For this review, take the finished solid that the model builds, in its own axes (mm). Give positions to 0.01 mm unless a question says otherwise; leave off trailing zeros. Loops run counter-clockwise (first coordinate to the right, second up) from the corner with the lowest first, then second, coordinate; pieces in that order, holes last. Notation, with made-up numbers: (-26.75, 21) - (-14.75, 21) arc R10 cw to (-14.75, 37) - close; hole circle Ø3 at (-23, 31.5). An arc over 180 degrees is marked (long way). Answer in a Markdown table with one row per item.
```python
from build123d import *

# Parameters (mm, degrees)
F0_W     = 21
F0_H     = 21
F1_DEPTH = 680
F3_DEPTH = 12.5


with BuildPart() as f1:
    # F0 (on Top) → F1 (new body)
    with BuildSketch(Plane.XY):
        with BuildLine():
            ThreePointArc((12.5, 9.5), (11.62132, 11.62132), (9.5, 12.5))
            Line((9.5, 12.5), (-9.5, 12.5))
            ThreePointArc((-9.5, 12.5), (-11.62132, 11.62132), (-12.5, 9.5))
            Line((-12.5, 9.5), (-12.5, -9.5))
            ThreePointArc((-12.5, -9.5), (-11.62132, -11.62132), (-9.5, -12.5))
            Line((-9.5, -12.5), (9.5, -12.5))
            ThreePointArc((9.5, -12.5), (11.62132, -11.62132), (12.5, -9.5))
            Line((12.5, -9.5), (12.5, 9.5))
        make_face()
        Rectangle(F0_W, F0_H, mode=Mode.SUBTRACT)
    extrude(amount=F1_DEPTH)

    # F2 (on Right) → F3 (cut, symmetric)
    with BuildSketch(Plane.YZ):
        Polygon((12.5, 25), (-12.5, 0), (12.5, 0), align=None)
        Polygon((-12.5, 650.5), (12.5, 625.5), (12.5, 680), (-12.5, 680), align=None)
    extrude(amount=F3_DEPTH, both=True, mode=Mode.SUBTRACT)


solid = f1.part
```
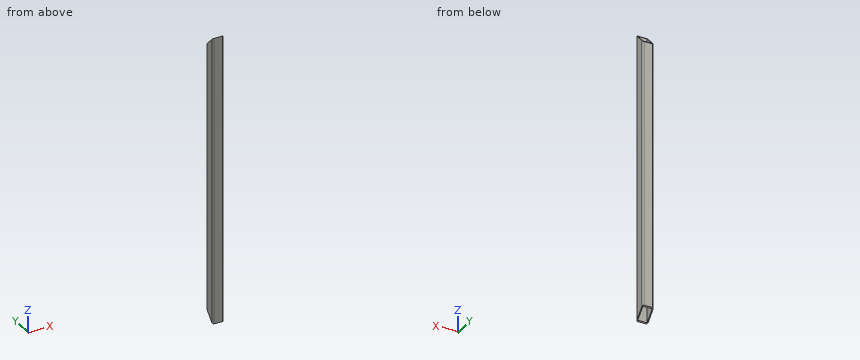
1. We need section C-C, the plane z = 149. Give the boundary of the cut face in (x, y).
Values:
| item | result |
|---|---|
| outline | (-12.5, -9.5) arc R3 ccw to (-9.5, -12.5) - (9.5, -12.5) arc R3 ccw to (12.5, -9.5) - (12.5, 9.5) arc R3 ccw to (9.5, 12.5) - (-9.5, 12.5) arc R3 ccw to (-12.5, 9.5) - close; hole (-10.5, -10.5) - (10.5, -10.5) - (10.5, 10.5) - (-10.5, 10.5) - close |
2. Wall thickness on line 1 (X direction, y = -9.25, z = 199.5); line 2 (X direction, y = -10.75, z = 553): over which ranges is each line inside the solid? List them lowest first. Write a range as [from, to].
Values:
| item | result |
|---|---|
| line 1 | x = [-12.5, -10.5], [10.5, 12.5] |
| line 2 | x = [-12.23, 12.23] |
3. We need section A-A, the plane y = 2.25. Give the boundary of the cut face in (x, z), and give its area (3 significant figures).
Values:
| item | result |
|---|---|
| outline | (-12.5, 14.75) - (-10.5, 14.75) - (-10.5, 635.75) - (-12.5, 635.75) - close; (10.5, 14.75) - (12.5, 14.75) - (12.5, 635.75) - (10.5, 635.75) - close |
| area | 2,480 mm^2 |
4. We need section B-B, the plane x = -1.75. Give the boundary of the cut face in (y, z), and give its area (3 significant figures).
Values:
| item | result |
|---|---|
| outline | (-12.5, 0) - (-10.5, 2) - (-10.5, 648.5) - (-12.5, 650.5) - close; (10.5, 23) - (12.5, 25) - (12.5, 625.5) - (10.5, 627.5) - close |
| area | 2,500 mm^2 |
